CAD build for the part. Positions are in the model's coordinates, mm. A direction names the side the tool comes from. Coordinates: 2 decimals unless noted, no trailing zeros. Order: outer loops, then holes, each group sorted by start corner. A loop starts at its lowest first (then second) coordinate and runs counter-clockwise, first axis right, second up. Notation, with made-up numbers: M 31,-23.75 L 73,-23.75 A21 ccw 73,-12.75 Z; hole C -13.5,41.25 d7. An arc over 180 degrees is marked long. One line per item, written item: value.
from build123d import *

# Parameters (mm, degrees)
SKETCH1_R               = 12.7
SKETCH1_R_2             = 10.5
BOSS_EXTRUDE1_DEPTH     = 71
BOSS_EXTRUDE2_DEPTH     = 63
CUT_EXTRUDE1_DEPTH      = 8
CUT_EXTRUDE2_DEPTH      = 15
CUT_EXTRUDE2_DEPTH_BACK = 16
SKETCH4_R               = 22.297733005
SKETCH5_R               = 2
CUT_EXTRUDE3_DEPTH      = 4
CUT_EXTRUDE4_START      = -4
SKETCH6_R               = 2
CUT_EXTRUDE4_DEPTH      = 4


with BuildPart() as part:
    # Sketch1 → Boss-Extrude1 (new body)
    with BuildSketch(Plane(origin=(0, 0, 0), x_dir=(1, 0, 0), z_dir=(0, 1, 0))):
        with Locations(Location((0, 0, 0), (0, 0, 270))):
            Circle(SKETCH1_R)
        with Locations(Location((0, 0, 0), (0, 0, 270))):
            Circle(SKETCH1_R_2, mode=Mode.SUBTRACT)
    extrude(amount=BOSS_EXTRUDE1_DEPTH)

    # Sketch2 → Boss-Extrude2 (add)
    with BuildSketch(Plane.XZ):
        with BuildLine():
            Line((12.7, 12.7), (0, 12.7))
            ThreePointArc((0, 12.7), (8.980256121, 8.980256121), (12.7, 0))
            Line((12.7, 0), (12.7, 12.7))
        make_face()
        with BuildLine():
            Line((12.7, -12.7), (12.7, 0))
            ThreePointArc((12.7, 0), (8.980256121, -8.980256121), (0, -12.7))
            Line((0, -12.7), (12.7, -12.7))
        make_face()
    extrude(amount=-BOSS_EXTRUDE2_DEPTH)

    # Sketch3 → Cut-Extrude1 (cut)
    with BuildSketch(Plane.XZ):
        with BuildLine():
            Line((12.7, 12.7), (0, 12.7))
            ThreePointArc((0, 12.7), (8.980256109, 8.980256133), (12.7, 3.4e-08))
            Line((12.7, 3.4e-08), (12.7, 12.7))
        make_face()
        with BuildLine():
            Line((12.7, -12.7), (12.7, 3.4e-08))
            ThreePointArc((12.7, 3.4e-08), (8.980256133, -8.980256109), (0, -12.7))
            Line((0, -12.7), (12.7, -12.7))
        make_face()
    extrude(amount=-CUT_EXTRUDE1_DEPTH, mode=Mode.SUBTRACT)

    # Sketch4 → Cut-Extrude2 (cut, two sides: drawn at the far end of the back side and taken through both)
    with BuildSketch(Plane.XY.offset(-CUT_EXTRUDE2_DEPTH_BACK)):
        with Locations((22.331187996, 35.5)):
            Circle(SKETCH4_R)
    extrude(amount=CUT_EXTRUDE2_DEPTH + CUT_EXTRUDE2_DEPTH_BACK, mode=Mode.SUBTRACT)

    # Sketch5 → Cut-Extrude3 (cut)
    with BuildSketch(Plane(origin=(0, 0, -12.7), x_dir=(-1, 0, 0), z_dir=(0, 0, -1))):
        with Locations((-8.7, 58.5)):
            Circle(SKETCH5_R)
        with Locations((-8.7, 12.5)):
            Circle(SKETCH5_R)
    extrude(amount=-CUT_EXTRUDE3_DEPTH, mode=Mode.SUBTRACT)

    # Sketch6 → Cut-Extrude4 (cut)
    with BuildSketch(Plane.XY.offset(12.7).offset(CUT_EXTRUDE4_START)):
        with Locations(Location((8.7, 58.5, 0), (0, 0, 180))):
            Circle(SKETCH6_R)
        with Locations(Location((8.7, 12.5, 0), (0, 0, 180))):
            Circle(SKETCH6_R)
    extrude(amount=CUT_EXTRUDE4_DEPTH, mode=Mode.SUBTRACT)


solid = part.part
Q1. Which spindle directions (+Z, -Z, +X, -X, +Y, -Y) get a long thin tool onto all of the face, cutting with end or side? Do faces 1 (the face through (7.625, 14.186, -10.728)), 2 (the face through (10, 8, -10)), 3 (the face through (7.625, 10.814, 10.672)), 4 (the face through (10, 63, -10)). Say none if no direction does.
Recorded:
face 1: -Z
face 2: -Z, +X, -Y
face 3: +Z
face 4: -Z, +X, +Y
Q2. Slice it at C-C (y = 58.5). List the corners of the cut face in (x, z), plus the area to 3 significant figures.
Recorded:
outline: M 0,-12.7 L 6.7,-12.7 L 6.7,-8.7 L 10.7,-8.7 L 10.7,-12.7 L 12.7,-12.7 L 12.7,12.7 L 10.7,12.7 L 10.7,8.7 L 6.7,8.7 L 6.7,12.7 L 0,12.7 A12.7 ccw Z; hole C 0,0 d21
area: 198 mm^2
Q3. Slice it at B-B (z = -3). List the corners of the cut face in (x, y).
Recorded:
outline: M -12.34,0 L -10.06,0 L -10.06,71 L -12.34,71 Z; M 10.06,0 L 12.34,0 L 12.34,8 L 12.7,8 L 12.7,15.39 A22.3 cw 10.06,16.88 Z; M 10.06,54.12 A22.3 cw 12.7,55.61 L 12.7,63 L 12.34,63 L 12.34,71 L 10.06,71 Z
Q4. Pin check, flat tips, straight feed: pin 1 Ø3 at (x, y) = (9, 58.5) entering from -Z; pin 2 Ø1.2 at (x, y) = (8.5, 12) entering from +Z; pin 3 Ø4 at (x, y) = (-8, 31.5) entering from -Z. Stop position of each tip, or through.
Recorded:
pin 1: stops at z = -8.7
pin 2: stops at z = 8.7
pin 3: stops at z = -11.19
Q5. Slice it at D-D (x = -6.75). List the corners of the cut face in (y, z).
Recorded:
outline: M 0,-10.76 L 71,-10.76 L 71,-8.04 L 0,-8.04 Z; M 0,8.04 L 71,8.04 L 71,10.76 L 0,10.76 Z
Q6. Mould opens along X. For faces 5 (the face through (8.96, 56.517, 10.672)), 6 (the face through (12.7, 12, 0)), 7 (the face through (10, 63, 10)) say: released by +X, released by -X, zero draft, split by the parting line, or undercut.
Recorded:
face 5: undercut
face 6: released by +X
face 7: zero draft
Q7. Slice it at A-A (x = 3.5). List the corners of the cut face in (y, z).
Recorded:
outline: M 0,-12.21 L 8,-12.21 L 8,-12.7 L 23.56,-12.7 L 23.56,-9.9 L 0,-9.9 Z; M 0,9.9 L 23.56,9.9 L 23.56,12.7 L 8,12.7 L 8,12.21 L 0,12.21 Z; M 47.44,-12.7 L 63,-12.7 L 63,-12.21 L 71,-12.21 L 71,-9.9 L 47.44,-9.9 Z; M 47.44,9.9 L 71,9.9 L 71,12.21 L 63,12.21 L 63,12.7 L 47.44,12.7 Z
Q8. Drill centre lines: line 1 along Y through (x, z) = (10, -10); line 2 along Y through (x, z) = (8.7, -10.7); line 3 along Z through (x, y) = (-9.75, 57.5). Where is each one in solid material? Low to high.
Recorded:
line 1: y = 8 to 10.98, 14.02 to 16.92, 54.08 to 56.98, 60.02 to 63
line 2: y = 8 to 10.5, 14.5 to 17.85, 53.15 to 56.5, 60.5 to 63
line 3: z = -8.14 to -3.9, 3.9 to 8.14
